Build history of the part. All positions in model axes, mm. A direction names the side the tool comes from. Round coordinates to 2 decimals unless told otherwise and drop trailing zeros. Write each loop counter-clockwise with the first axis right and the second up, starting at its lowest first coordinate (ties: lowest second). Pieces come first, ordered by that corner, then holes.
1) Flat gauge pins, fed straight in: pin 1 (5 mm diameter, centred on x = 26.17, y = -56.83, fed in from -Z); pin 2 (1 mm diameter, centred on y = -116.5, z = 1, fed in from -X); pin 3 (1.9 mm diameter, centred on x = 16, y = -136, fed in from +Z). Where does each tip first touch, or does it go through?
2) Which spindle directions (+Z, -Z, +X, -X, +Y, -Y) get a long thin tool onto all of the face, cutting with end or side? Do faces 1 (the flat face through (31, -53, 1)), 2 (the cylindrical face through (18.797, -130.859, 1.014)), 3 (the cylindrical face through (16, -87, 1)), 4 (the flat face through (16, -54, 1)), 5 (the flat face through (28, -95, 1)). Say none if no direction does.
3) Wall check: probe 1 along X at (y, z) = (-73.5, 0.15); probe 2 along Y at (x, z) = (25, 1.95); probe 3 along X at (y, z) = (-104, 0.55). Give the ranges that are in metal, low to high.
4) Saw through at B-B (x = 31.5). Write the cut outline in (y, z).
5) Saw through at C-C (y = -116.5). Write the cut outline in (x, z), plus the area to 3 significant figures.
6) Saw through at D-D (z = 1). State how many separate pieces and enclosed holes the cut face has, plus the area to 3 significant figures.
7) Pull direction Y, two halves, no side cores. Call faces 6 (the cylindrical face through (16, -58.8, 1)), 7 (the cylindrical face through (32.85, -55.07, 1.01)), 8 (the flat face through (22, -140, 1)): +Y half, -Y half, draft (parallel to the pull), parting line (faces both ways), or undercut.
8) Saw through at A-A (y = -84). Write the cut outline in (x, z).
from build123d import *

# Parameters (mm, degrees)
SKETCH1_R           = 1.6
BOSS_EXTRUDE1_DEPTH = 2
FILLET1_R           = 4
FILLET2_R           = 2


with BuildPart() as part:
    # Sketch1 → Boss-Extrude1 (new body)
    with BuildSketch(Plane.XY):
        Polygon((28, -126.339745962), (28, -63.660254038), (33, -58.660254038), (33, -55), (28, -50), (20, -50), (12, -58), (12, -87.8), (20, -95.8), (20, -132), (12, -132), (12, -140), (28, -140), (33, -135), (33, -131.339745962), align=None)
        with Locations((26.169872981, -133.169872981)):
            Circle(SKETCH1_R, mode=Mode.SUBTRACT)
        with Locations((26.169872981, -56.830127019)):
            Circle(SKETCH1_R, mode=Mode.SUBTRACT)
        with Locations((16, -136)):
            Circle(SKETCH1_R, mode=Mode.SUBTRACT)
        with BuildLine():
            Line((17.6, -85.4), (17.6, -60.4))
            ThreePointArc((17.6, -60.4), (16, -58.8), (14.4, -60.4))
            Line((14.4, -60.4), (14.4, -85.4))
            ThreePointArc((14.4, -85.4), (16, -87), (17.6, -85.4))
        make_face(mode=Mode.SUBTRACT)
    extrude(amount=BOSS_EXTRUDE1_DEPTH)

    # Fillet1
    fillet1_edges = [part.edges().sort_by_distance(p)[0] for p in [
        (12, -140, 1),
        (20, -132, 1),
        (12, -132, 1),
    ]]
    fillet(fillet1_edges, radius=FILLET1_R - 0.0001)  # a hair under: the kernel refuses the full size

    # Fillet2
    fillet2_edges = [part.edges().sort_by_distance(p)[0] for p in [
        (33, -131.339745962, 1),
        (33, -135, 1),
        (28, -140, 1),
        (20, -95.8, 1),
        (12, -87.8, 1),
        (12, -58, 1),
        (20, -50, 1),
        (28, -50, 1),
        (33, -55, 1),
        (33, -58.660254038, 1),
        (28, -63.660254038, 1),
        (28, -126.339745962, 1),
    ]]
    fillet(fillet2_edges, radius=FILLET2_R)


solid = part.part
Evaluation:
1. pin 1: stops at z = 0
1. pin 2: stops at x = 20
1. pin 3: passes through
2. face 1: +Z, -Z, +X, +Y
2. face 2: +Z, -Z, -X
2. face 3: +Z, -Z
2. face 4: +Z, -Z, -X, +Y
2. face 5: +Z, -Z, +X
3. probe 1: x = 12 to 14.4, 17.6 to 28
3. probe 2: y = -140 to -134.26, -132.08 to -57.92, -55.74 to -50
3. probe 3: x = 20 to 28
4. outline: (-136.5, 0) - (-129.84, 0) - (-129.84, 2) - (-136.5, 2) - close; (-60.16, 0) - (-53.5, 0) - (-53.5, 2) - (-60.16, 2) - close
5. outline: (20, 0) - (28, 0) - (28, 2) - (20, 2) - close
5. area: 16.0 mm2
6. separate pieces: 1
6. enclosed holes: 4
6. area: 1,060 mm2
7. face 6: undercut
7. face 7: +Y half
7. face 8: -Y half
8. outline: (12, 0) - (14.4, 0) - (14.4, 2) - (12, 2) - close; (17.6, 0) - (28, 0) - (28, 2) - (17.6, 2) - close
